Could you check a few things on this drawing? It's one solid part, dimensions in mm from its lowest x, y, z. A direction names the side the tool comes from. Give positions to 0.01 mm unless a question says otherwise; leave off trailing zeros. Loops run counter-clockwise (first coordinate to the right, second up) from the corner with the lowest first, then second, coordinate; pieces in that order, holes last. Notation, with made-up numbers: M 66.5,34 L 100.5,34 A9 cw 100.5,39 Z; hole C -32,7.5 d9. An arc over 180 degrees is marked long. Answer in a Markdown table with one row per item. Add a question column.
1. If we section it at C-C on x = 39: List the corners of the cut face in (y, z) for me, then the cut area to 3 significant figures.
2. If we section it at A-A on y = 8.89: List the corners of the cut face in (x, z) for me.
3. I need wall thicknesses on line 1 along Y through (x, z) = (31.75, 36.25); line 2 along Z through (x, y) = (57.5, 8.89); line 3 along Y through (x, z) = (26.5, 53). Which ranges of each line are inside material? Lowest first, please. Write a range as from..to.
4. Which directions (+Z, -Z, +X, -X, +Y, -Y) give clear straight access to the entire face, cutting with the end or side of a thin tool? Please do the marked faces 1, 2, 3 and 4.
5. I'm going to push flat-ended pins straight in: pin 1 Ø1 at (x, y) = (19.5, 10) entering from -Z; pin 2 Ø6 at (y, z) = (3, 48) entering from +X; pin 3 Ø10.5 at (y, z) = (8.89, 31.75) entering from +X; pin 4 Ø3 at (x, z) = (41.5, 25.5) entering from +Y. Where does each tip first touch, or does it pass through?
6. If we section it at B-B on z = 34: List the corners of the cut face in (x, y) for me, then the cut area to 3 significant figures.
7. If we section it at D-D on z = 24: List the corners of the cut face in (x, y) for me, then the cut area to 3 significant figures.
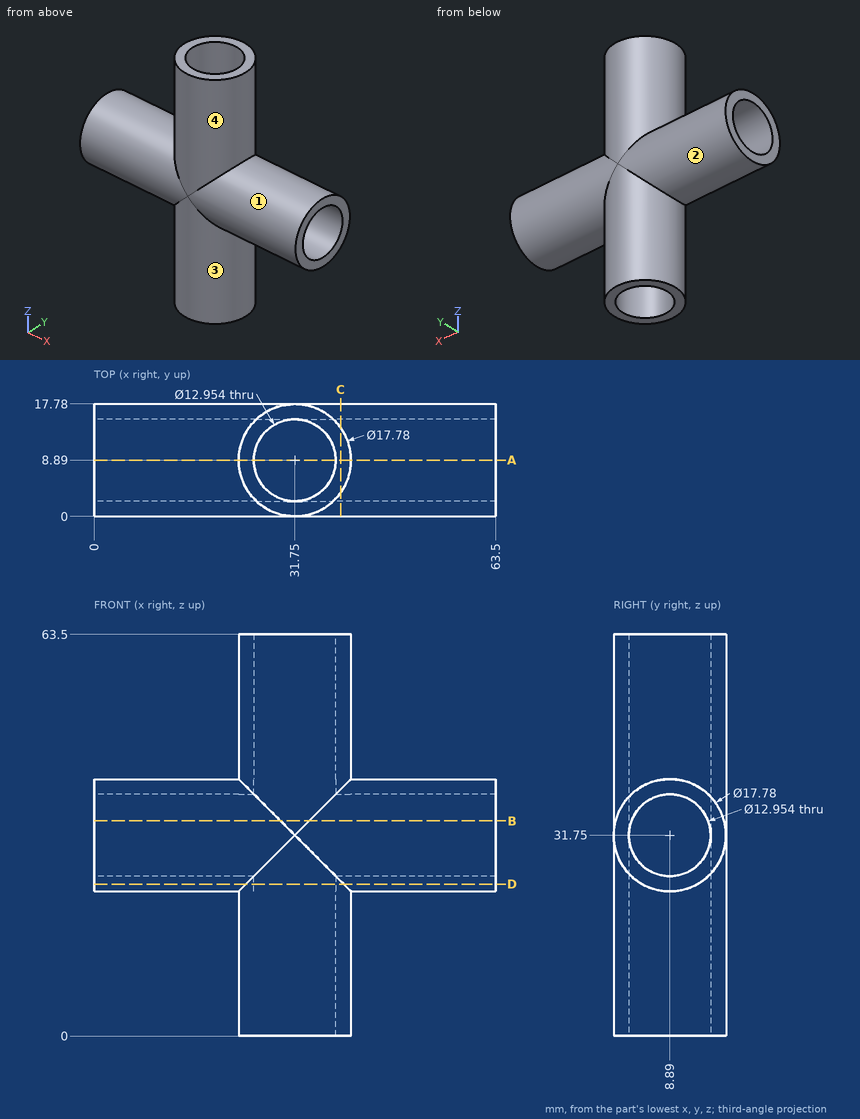
Results:
| question | item | result |
|---|---|---|
| 1 | outline | M 3.75,0 L 14.03,0 L 14.03,24.5 A8.89 ccw 14.03,39 L 14.03,63.5 L 3.75,63.5 L 3.75,39 A8.89 ccw 3.75,24.5 Z; hole C 8.89,31.75 d12.95 |
| 1 | area | 598 mm2 |
| 2 | outline | M 0,22.86 L 22.86,22.86 L 22.86,0 L 25.27,0 L 25.27,25.27 L 0,25.27 Z; M 0,38.23 L 25.27,38.23 L 25.27,63.5 L 22.86,63.5 L 22.86,40.64 L 0,40.64 Z; M 38.23,0 L 40.64,0 L 40.64,22.86 L 63.5,22.86 L 63.5,25.27 L 38.23,25.27 Z; M 38.23,38.23 L 63.5,38.23 L 63.5,40.64 L 40.64,40.64 L 40.64,63.5 L 38.23,63.5 Z |
| 3 | line 1 | 0..2.41, 15.37..17.78 |
| 3 | line 2 | 22.86..25.27, 38.23..40.64 |
| 3 | line 3 | 1.72..5.1, 12.68..16.06 |
| 4 | face 1 | +X |
| 4 | face 2 | -X |
| 4 | face 3 | -Z |
| 4 | face 4 | +Z |
| 5 | pin 1 | z = 22.88 |
| 5 | pin 2 | x = 40.16 |
| 5 | pin 3 | through |
| 5 | pin 4 | y = 16.4 |
| 6 | outline | M 0,0.29 L 29.5,0.29 A8.89 ccw 34,0.29 L 63.5,0.29 L 63.5,2.82 L 34,2.82 A6.48 cw 29.5,2.82 L 0,2.82 Z; M 0,14.96 L 29.5,14.96 A6.48 cw 34,14.96 L 63.5,14.96 L 63.5,17.49 L 34,17.49 A8.89 ccw 29.5,17.49 L 0,17.49 Z |
| 6 | area | 320 mm2 |
| 7 | outline | M 0,4.53 L 24,4.53 A8.89 ccw 39.5,4.53 L 63.5,4.53 L 63.5,13.25 L 39.5,13.25 A8.89 ccw 24,13.25 L 0,13.25 Z; hole C 31.75,8.89 d12.95 |
| 7 | area | 521 mm2 |
